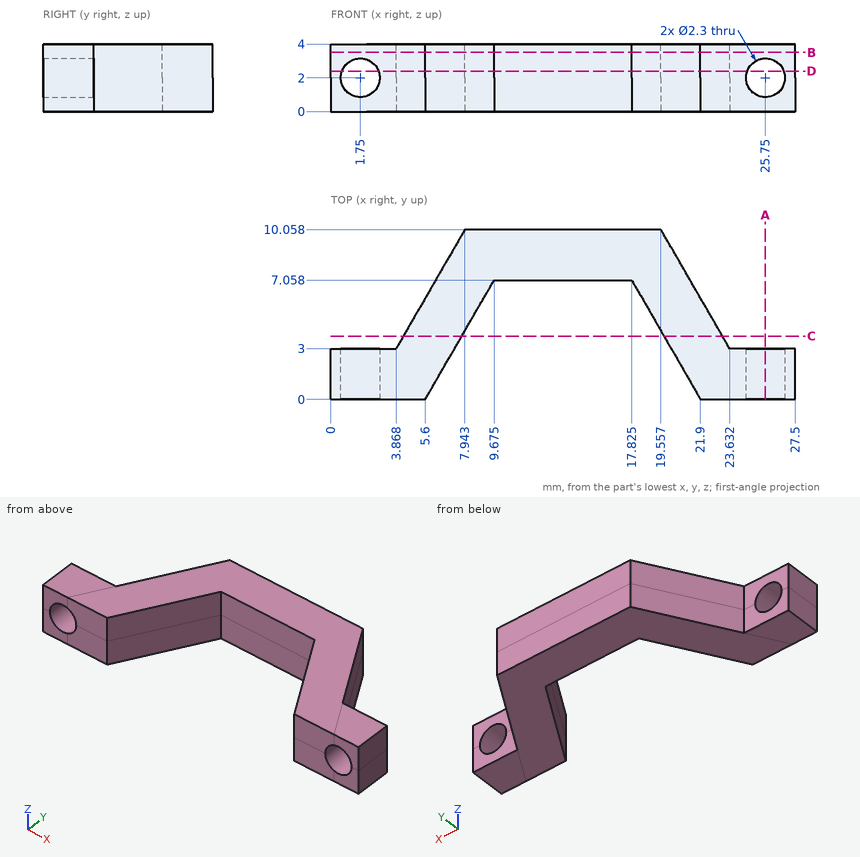
Geometry check sheet. Reference: drawing and pictorial views, mm from the part's lowest x, y, z. Give positions to 0.01 mm unless a question says otherwise; leave off trailing zeros. Loops run counter-clockwise (first coordinate to the right, second up) from the corner with the lowest first, then second, coordinate; pieces in that order, holes last.
1. Section check B-B, the plane z = 3.5. Enter the section's corners in (x, y) (3 decimals).
2. Thickness scan on line 1 (Z direction, x = 25.75, y = 1.85); line 2 (X direction, y = 2, z = 2) (1 decimal); line 3 (X direction, y = 1.9, z = 2). Record the ranges inside material, lowest first.
3. Section check C-C, the plane y = 3.75. Enter the section's corners in (x, z) (3 decimals), then the cut area to 3 significant figures.
4. Section check A-A, the plane x = 25.75. Enter the section's corners in (y, z), then the cut area to 3 significant figures.
5. Go/stop test with flat-tipped pins: pin 1 Ø0.6 at (x, z) = (13, 1.5) entering from -Y; pin 2 Ø2 at (x, z) = (25, 3) entering from +Y. Record where each tip stops, or that it passes through.
6. Section check D-D, the plane z = 2.4. Enter the section's corners in (x, y) (3 decimals).
Geometry says:
1. outline: (0, 0) - (5.6, 0) - (9.675, 7.058) - (17.825, 7.058) - (21.9, 0) - (27.5, 0) - (27.5, 3) - (23.632, 3) - (19.557, 10.058) - (7.943, 10.058) - (3.868, 3) - (0, 3) - close
2. line 1: z = 0 to 0.85, 3.15 to 4
2. line 2: x = 0 to 0.6, 2.9 to 6.8, 20.7 to 24.6, 26.9 to 27.5
2. line 3: x = 0 to 0.6, 2.9 to 6.7, 20.8 to 24.6, 26.9 to 27.5
3. outline: (4.301, 0) - (7.765, 0) - (7.765, 4) - (4.301, 4) - close; (19.735, 0) - (23.199, 0) - (23.199, 4) - (19.735, 4) - close
3. area: 27.7 mm2
4. outline: (0, 0) - (3, 0) - (3, 0.85) - (0, 0.85) - close; (0, 3.15) - (3, 3.15) - (3, 4) - (0, 4) - close
4. area: 5.10 mm2
5. pin 1: stops at y = 7.06
5. pin 2: stops at y = 3
6. outline: (0, 0) - (0.672, 0) - (0.672, 3) - (0, 3) - close; (2.828, 0) - (5.6, 0) - (9.675, 7.058) - (17.825, 7.058) - (21.9, 0) - (24.672, 0) - (24.672, 3) - (23.632, 3) - (19.557, 10.058) - (7.943, 10.058) - (3.868, 3) - (2.828, 3) - close; (26.828, 0) - (27.5, 0) - (27.5, 3) - (26.828, 3) - close
